Job drawing, mm, ordinate dimensions from the low corner. One solid piece. Round coordinates to 2 decimals unless told otherwise and drop trailing zeros. Loops run counter-clockwise (first coordinate to the right, second up) from the corner with the lowest first, then second, coordinate; pieces in that order, holes last. Notation, with made-up numbers: M 0,25 L 21,25 A26 ccw 21,42 Z; hole C -15,55.5 d7. An arc over 180 degrees is marked long. One line per item, written item: value.
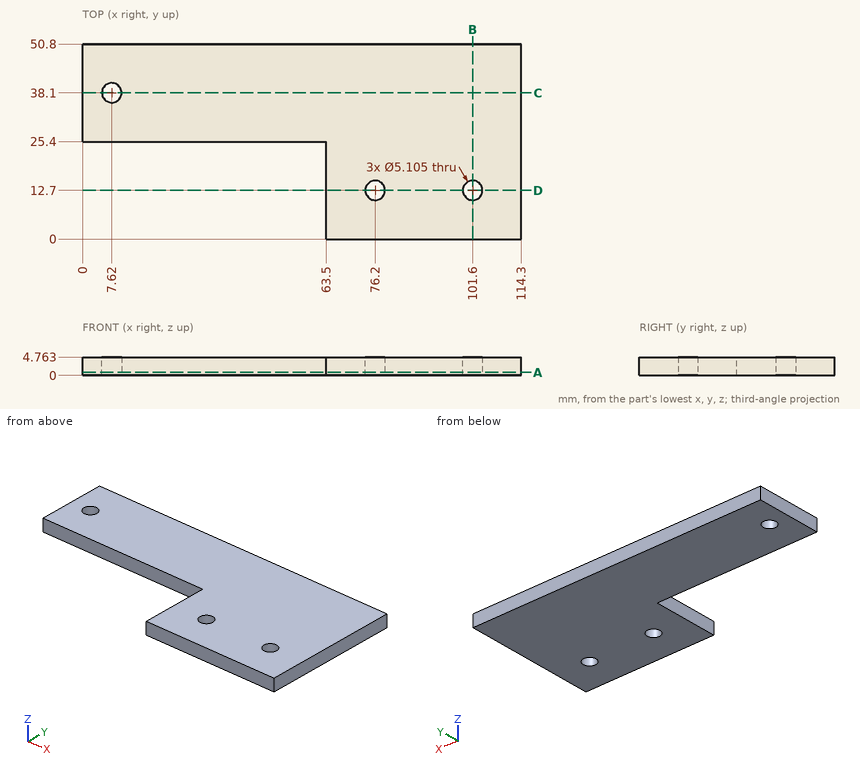
Item 1: Slice it at C-C, the plane y = 38.1. Give the cut face in (x, z).
Check values:
outline: M 0,0 L 5.07,0 L 5.07,4.76 L 0,4.76 Z; M 10.17,0 L 114.3,0 L 114.3,4.76 L 10.17,4.76 Z
Item 2: Slice it at A-A, the plane z = 0.8. Give the cut face in (x, y) (1 decimal).
Check values:
outline: M 0,25.4 L 63.5,25.4 L 63.5,0 L 114.3,0 L 114.3,50.8 L 0,50.8 Z; hole C 7.6,38.1 d5.1; hole C 76.2,12.7 d5.1; hole C 101.6,12.7 d5.1
Item 3: Wall check: line 1 along X through (y, z) = (12.7, 1.7); line 2 along X through (y, z) = (14, 2.65) (1 decimal); line 3 along Y through (x, z) = (101.6, 2). Give the ranges that are in metal, low to high.
Check values:
line 1: x = 63.5 to 73.65, 78.75 to 99.05, 104.15 to 114.3
line 2: x = 63.5 to 74, 78.4 to 99.4, 103.8 to 114.3
line 3: y = 0 to 10.15, 15.25 to 50.8
Item 4: Slice it at D-D, the plane y = 12.7. Give the cut face in (x, z).
Check values:
outline: M 63.5,0 L 73.65,0 L 73.65,4.76 L 63.5,4.76 Z; M 78.75,0 L 99.05,0 L 99.05,4.76 L 78.75,4.76 Z; M 104.15,0 L 114.3,0 L 114.3,4.76 L 104.15,4.76 Z
Item 5: Slice it at B-B, the plane x = 101.6. Give the cut face in (y, z).
Check values:
outline: M 0,0 L 10.15,0 L 10.15,4.76 L 0,4.76 Z; M 15.25,0 L 50.8,0 L 50.8,4.76 L 15.25,4.76 Z
Item 6: Drop flat-ended pins along their axis: P1, Ø6.5, axis at x = 76.2, y = 12.7, coming from the -Z side; P2, Ø1.4, axis at x = 40, z = 2, coming from the -Y side; P3, Ø1.4, axis at y = 16.5, z = 3, coming from the -X side; P4, Ø3, axis at x = 7.62, y = 38.1, coming from the -Z side. Give the stop position or say it passes through.
Check values:
P1: stops at z = 0
P2: stops at y = 25.4
P3: stops at x = 63.5
P4: passes through
